```python
from build123d import *

# Parameters (mm, degrees)
SKETCH_2_R               = 2
SKETCH_2_R_2             = 3
EXTRUDE_1_DEPTH          = 80
CUT_EXTRUDE_2_REACH      = 221.122
CUT_EXTRUDE_2_END_RADIUS = 55.2
SKETCH_6_W               = 15
SKETCH_6_H               = 20
SKETCH_7_W               = 50
SKETCH_7_H               = 20
CUT_EXTRUDE_3_DEPTH      = 265.578124336
CUT_EXTRUDE_4_REACH      = 221.122
CUT_EXTRUDE_4_END_RADIUS = 55
SKETCH_8_W               = 15
SKETCH_8_H               = 20
SKETCH_9_W               = 50
SKETCH_9_H               = 10
EXTRUDE_2_DEPTH          = 20


with BuildPart() as part:
    # Эскиз2 → Бобышка-Вытянуть1 (new body)
    with BuildSketch(Plane(origin=(0, 0, 0), x_dir=(0, 0, -1), z_dir=(1, 0, 0))):
        with BuildLine():
            Line((-47.804602289, 27.6), (-67.804602289, 27.6))
            Line((-67.804602289, 27.6), (-67.804602289, 95.2))
            Line((-67.804602289, 95.2), (197.773522047, 95.2))
            Line((197.773522047, 95.2), (197.773522047, 27.6))
            Line((197.773522047, 27.6), (177.773522047, 27.6))
            ThreePointArc((177.773522047, 27.6), (161.886250902, 44.955327869), (140.2, 54.083269132))
            Line((140.2, 54.083269132), (140.2, 45.2))
            Line((140.2, 45.2), (120.2, 45.2))
            Line((120.2, 45.2), (120.2, 54.083269132))
            ThreePointArc((120.2, 54.083269132), (98.513749098, 44.955327869), (82.626477953, 27.6))
            Line((82.626477953, 27.6), (47.804602289, 27.6))
            ThreePointArc((47.804602289, 27.6), (31.83374449, 45.096038759), (10, 54.286646609))
            Line((10, 54.286646609), (10, 45.2))
            Line((10, 45.2), (-10, 45.2))
            Line((-10, 45.2), (-10, 54.286646609))
            ThreePointArc((-10, 54.286646609), (-31.83374449, 45.096038759), (-47.804602289, 27.6))
        make_face()
        with Locations((-47.804602289, 85.2)):
            Circle(SKETCH_2_R, mode=Mode.SUBTRACT)
        with Locations((-57.804602289, 85.2)):
            Circle(SKETCH_2_R, mode=Mode.SUBTRACT)
        with Locations((90.2, 85.2)):
            Circle(SKETCH_2_R_2, mode=Mode.SUBTRACT)
        with Locations((167.7, 85.2)):
            Circle(SKETCH_2_R_2, mode=Mode.SUBTRACT)
    extrude(amount=EXTRUDE_1_DEPTH)

    # Вырез-Вытянуть2: up to this cylinder (the profile starts inside it)
    cut_extrude_2_end = Plane(origin=(40, 0, 0), z_dir=(-1, 0, 0)) * Cylinder(CUT_EXTRUDE_2_END_RADIUS, 618.644, mode=Mode.PRIVATE)
    # Эскиз6 → Вырез-Вытянуть2 (cut, up to the surface)
    with BuildSketch(Plane.XZ.offset(-45.2), mode=Mode.PRIVATE) as cut_extrude_2_sk1:
        with Locations((7.5, 0)):
            Rectangle(SKETCH_6_W, SKETCH_6_H)
    cut_extrude_2_tool1 = extrude(cut_extrude_2_sk1.sketch, amount=-CUT_EXTRUDE_2_REACH, mode=Mode.PRIVATE) & cut_extrude_2_end
    add(cut_extrude_2_tool1.solids().sort_by_distance((7.5, 45.2, 0))[0], mode=Mode.SUBTRACT)
    # Эскиз6 → Вырез-Вытянуть2 (cut, up to the surface)
    with BuildSketch(Plane.XZ.offset(-45.2), mode=Mode.PRIVATE) as cut_extrude_2_sk2:
        with Locations((72.5, 0)):
            Rectangle(SKETCH_6_W, SKETCH_6_H)
    cut_extrude_2_tool2 = extrude(cut_extrude_2_sk2.sketch, amount=-CUT_EXTRUDE_2_REACH, mode=Mode.PRIVATE) & cut_extrude_2_end
    add(cut_extrude_2_tool2.solids().sort_by_distance((72.5, 45.2, 0))[0], mode=Mode.SUBTRACT)

    # Эскиз7 → Вырез-Вытянуть3 (cut)
    with BuildSketch(Plane(origin=(0, 0, -197.773522047), x_dir=(-1, 0, 0), z_dir=(0, 0, -1))):
        with Locations((-40, 85.2)):
            Rectangle(SKETCH_7_W, SKETCH_7_H)
    extrude(amount=-CUT_EXTRUDE_3_DEPTH, mode=Mode.SUBTRACT)

    # Вырез-Вытянуть4: up to this cylinder (the profile starts inside it)
    cut_extrude_4_end = Plane(origin=(40, 0, -130.2), z_dir=(-1, 0, 0)) * Cylinder(CUT_EXTRUDE_4_END_RADIUS, 618.244, mode=Mode.PRIVATE)
    # Эскиз8 → Вырез-Вытянуть4 (cut, up to the surface)
    with BuildSketch(Plane.XZ.offset(-45.2), mode=Mode.PRIVATE) as cut_extrude_4_sk1:
        with Locations((7.5, -130.2)):
            Rectangle(SKETCH_8_W, SKETCH_8_H)
    cut_extrude_4_tool1 = extrude(cut_extrude_4_sk1.sketch, amount=-CUT_EXTRUDE_4_REACH, mode=Mode.PRIVATE) & cut_extrude_4_end
    add(cut_extrude_4_tool1.solids().sort_by_distance((7.5, 45.2, -130.2))[0], mode=Mode.SUBTRACT)
    # Эскиз8 → Вырез-Вытянуть4 (cut, up to the surface)
    with BuildSketch(Plane.XZ.offset(-45.2), mode=Mode.PRIVATE) as cut_extrude_4_sk2:
        with Locations((72.5, -130.2)):
            Rectangle(SKETCH_8_W, SKETCH_8_H)
    cut_extrude_4_tool2 = extrude(cut_extrude_4_sk2.sketch, amount=-CUT_EXTRUDE_4_REACH, mode=Mode.PRIVATE) & cut_extrude_4_end
    add(cut_extrude_4_tool2.solids().sort_by_distance((72.5, 45.2, -130.2))[0], mode=Mode.SUBTRACT)

    # Эскиз9 → Бобышка-Вытянуть2 (add)
    with BuildSketch(Plane(origin=(0, 75.2, 0), x_dir=(1, 0, 0), z_dir=(0, 1, 0))):
        with Locations((40, 25.2)):
            Rectangle(SKETCH_9_W, SKETCH_9_H)
    extrude(amount=EXTRUDE_2_DEPTH)


solid = part.part
```
CAD build for the part. Positions are in the model's coordinates, mm. A direction names the side the tool comes from. Round coordinates to 2 decimals unless told otherwise and drop trailing zeros. Order: outer loops, then holes, each group sorted by start corner. A loop starts at its lowest first (then second) coordinate and runs counter-clockwise, first axis right, second up. Notation, with made-up numbers: (-24.5, 13.5) - (5.5, 13.5) arc R20 cw to (5.5, 45.5) - close; hole circle Ø9 at (-10.5, -37). An arc over 180 degrees is marked (long way). Answer as CSV lines item,"result". Start each with the question number.
1. Saw through at A-A, the plane x = 9.5. Write the cut outline in (y, z).
2. Tool access for faces 4 (the face through (15, 50, -130)), 5 (the face through (15, 85, -115)), 6 (the face through (40, 50, 10)), 7 (the face through (40, 85, -20.2)): list every direction of +Z, -Z, +X, -X, +Y, -Y with a clear straight run to the whole face (end or side of a thin tool).
3. Pull direction X, two halves, no side cores. Call faces 1 (the face through (0, 69, -67)), 2 (the face through (15, 85, 23)), 3 (the face through (39, 27.6, 58)): +X half, -X half, draft (parallel to the pull), parting line (faces both ways), or undercut.
4. Drill centre lines: L1, parallel to Z at x = 11, y = 85; L2, parallel to X at y = 90.5, z = 31; L3, parallel to Y at x = 72, z = 48. Where is each one in solid material? Low to high. Write a range as [from, to].
5. Saw through at D-D, the plane x = 60. Write the cut outline in (y, z).
6. Saw through at B-B, the plane z = -167.7. Write the cut outline in (x, y), and give its area (3 significant figures).
7. Pin check, flat tips, straight feed: pin 1 (25 mm diameter, centred on x = 28, z = -127, fed in from +Y); pin 2 (3 mm diameter, centred on y = 51, z = 1, fed in from +X); pin 3 (5 mm diameter, centred on x = 21.5, z = -105.5, fed in from -Y); pin 4 (5.5 mm diameter, centred on y = 85.2, z = -90.2, fed in from +X). Stop position of each tip, or through.
8. Saw through at C-C, the plane y = 34. Write the cut outline in (x, z).
Model answer:
1,outline,"(27.6, -197.77) - (95.2, -197.77) - (95.2, 67.8) - (27.6, 67.8) - (27.6, 47.8) arc R55.2 cw to (27.6, -47.8) - (27.6, -82.63) arc R55 cw to (27.6, -177.77) - close; hole circle Ø6 at (85.2, -167.7); hole circle Ø6 at (85.2, -90.2); hole circle Ø4 at (85.2, 47.8); hole circle Ø4 at (85.2, 57.8)"
2,face 4,"-X, -Y"
2,face 5,"-Z, +Y"
2,face 6,"+X, -X, -Y"
2,face 7,"+Z, +Y"
3,face 1,"-X half"
3,face 2,"undercut"
3,face 3,"draft"
4,L1,"z = [-197.77, -170.69], [-164.71, -93.19], [-87.21, 45.81], [49.79, 55.81], [59.79, 67.8]"
4,L2,"x = [0, 15], [65, 80]"
4,L3,"y = [27.6, 83.21], [87.19, 95.2]"
5,outline,"(27.6, -197.77) - (75.2, -197.77) - (75.2, -30.2) - (95.2, -30.2) - (95.2, -20.2) - (75.2, -20.2) - (75.2, 67.8) - (27.6, 67.8) - (27.6, 47.8) arc R55.2 cw to (54.29, 10) - (45.2, 10) - (45.2, -10) - (54.29, -10) arc R55.2 cw to (27.6, -47.8) - (27.6, -82.63) arc R55 cw to (54.08, -120.2) - (45.2, -120.2) - (45.2, -140.2) - (54.08, -140.2) arc R55 cw to (27.6, -177.77) - close"
6,outline,"(0, 40.23) - (80, 40.23) - (80, 82.2) - (65, 82.2) - (65, 75.2) - (15, 75.2) - (15, 82.2) - (0, 82.2) - close; (0, 88.2) - (15, 88.2) - (15, 95.2) - (0, 95.2) - close; (65, 88.2) - (80, 88.2) - (80, 95.2) - (65, 95.2) - close"
6,area,"3,220 mm²"
7,pin 1,"stops at y = 75.2"
7,pin 2,"stops at x = 65"
7,pin 3,"stops at y = 47.8"
7,pin 4,"passes through"
8,outline,"(0, -197.77) - (80, -197.77) - (80, -173.43) - (0, -173.43) - close; (0, -86.97) - (80, -86.97) - (80, -43.49) - (0, -43.49) - close; (0, 43.49) - (80, 43.49) - (80, 67.8) - (0, 67.8) - close"
